Geometry check sheet. Reference: the model listing, model coordinates, mm. Face numbers are marked on the shaded views. A direction names the side the tool comes from. Give positions to 0.01 mm unless a question says otherwise; leave off trailing zeros. Write each loop counter-clockwise with the first axis right and the second up, starting at its lowest first coordinate (ties: lowest second). Pieces come first, ordered by that corner, then holes. Notation, with made-up numbers: M -6,28 L 24,28 A25 ccw 24,42 Z; hole C -9.5,85.25 d4. An arc over 180 degrees is marked long. Write each question's results on one line, items separated by ' | '.
```python
from build123d import *

# Parameters (mm, degrees)
SKETCH019_W             = 83
SKETCH019_H             = 28
SKETCH019_W_2           = 79
SKETCH019_H_2           = 24
REVOLUTION_ANGLE        = 35
SKETCH020_W             = 83
SKETCH020_H             = 28
SKETCH020_W_2           = 79
SKETCH020_H_2           = 24
PAD010_DEPTH            = 60
POCKET006_DEPTH         = 83.001
SKETCH022_W             = 83
SKETCH022_H             = 28
SKETCH022_W_2           = 79
SKETCH022_H_2           = 24
PAD011_DEPTH            = 15
BODY005_PLACEMENT_ANGLE = 180


with BuildPart() as part:
    # Sketch019 → Revolution (revolve)
    with BuildSketch(Plane(origin=(310, 156, 1), x_dir=(0, 1, 0), z_dir=(1, 0, 0))):
        with Locations((41.5, 14)):
            Rectangle(SKETCH019_W, SKETCH019_H)
        with Locations((41.5, 14)):
            Rectangle(SKETCH019_W_2, SKETCH019_H_2, mode=Mode.SUBTRACT)
    revolve(axis=Axis((310, 156, 1), (0, 1, 0)), revolution_arc=REVOLUTION_ANGLE)

    # Sketch020 (on Face9 of Revolution) → Pad010 (new body)
    with BuildSketch(Plane(origin=(207.543276, 0, -145.323366), x_dir=(0, 1, 0), z_dir=(0.819152, 0, -0.573576))):
        with Locations((197.5, 192.627847)):
            Rectangle(SKETCH020_W, SKETCH020_H)
        with Locations((197.5, 192.627847)):
            Rectangle(SKETCH020_W_2, SKETCH020_H_2, mode=Mode.SUBTRACT)
    extrude(amount=PAD010_DEPTH)

    # Sketch021 (on Face11 of Pad010) → Pocket006 (cut, through all)
    with BuildSketch(Plane(origin=(0, 156, 0), x_dir=(0, 0, -1), z_dir=(0, -1, 0))):
        Polygon((21.946458, 367.179193), (33.414586, 359.149123), (25.384516, 347.680994), align=None)
    extrude(amount=-POCKET006_DEPTH, mode=Mode.SUBTRACT)

    # Sketch022 (on Face4 of Pocket006) → Pad011 (join)
    with BuildSketch(Plane(origin=(310, 0, 0), x_dir=(0, 1, 0), z_dir=(-1, 0, 0))):
        with Locations((197.5, -15)):
            Rectangle(SKETCH022_W, SKETCH022_H)
        with Locations((197.5, -15)):
            Rectangle(SKETCH022_W_2, SKETCH022_H_2, mode=Mode.SUBTRACT)
    extrude(amount=PAD011_DEPTH)


with BuildPart() as part_1:
    # Body005 placement: moved
    add(part.part.moved(Location((0, 395, 30))).rotate(Axis((0, 395, 30), (1, 0, 0)), BODY005_PLACEMENT_ANGLE))


solid = part_1.part
```
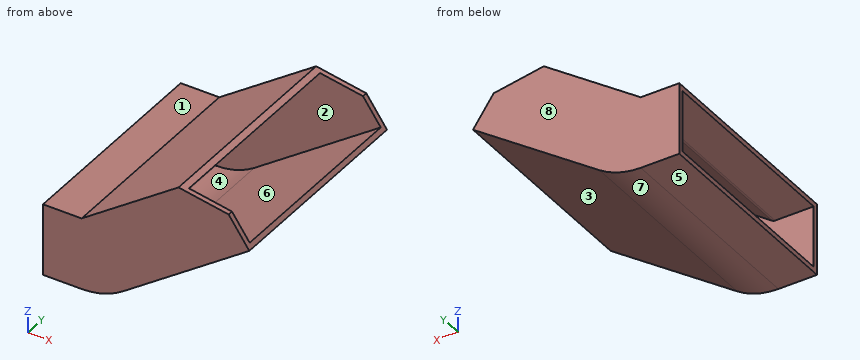
Q1. Section check C-C (z = 37.5). Enter the section's corners in (x, y).
Answer key:
outline: M 322.14,156 L 370.96,156 L 370.96,239 L 322.14,239 Z; hole M 325.63,158 L 367.47,158 L 367.47,237 L 325.63,237 Z
Q2. Access from +Z, -Z, +X, -X, +Y, -Y to the whole of each face (thin tool, end or side, straight path). Record for the marked faces 1, 2, 3, 4 and 5.
Answer key:
face 1: +Z, -X, +Y, -Y | face 2: none | face 3: -Z, +X, +Y, -Y | face 4: -X | face 5: -Z, +X, -X, +Y, -Y
Q3. Section check D-D (x = 368.5). Enter the section's corners in (y, z).
Answer key:
outline: M 156,35.78 L 239,35.78 L 239,50.06 L 237,50.06 L 237,38.22 L 158,38.22 L 158,50.06 L 156,50.06 Z
Q4. Release check for a two-part mould opening along X. For the marked faces 6, 7 and 8 record: released by +X, released by -X, zero draft, split by the parting line, or undercut.
Answer key:
face 6: undercut | face 7: released by +X | face 8: zero draft
Q5. Section check A-A (y = 191). Enter the section's corners in (x, z).
Answer key:
outline: M 295,1 L 310,1 A28 ccw 326.06,6.06 L 375.21,40.48 L 374.06,42.12 L 324.91,7.7 A26 cw 310,3 L 295,3 Z; M 295,27 L 310,27 A2 ccw 311.15,27.36 L 350.47,54.89 L 347.68,55.38 L 310,29 L 295,29 Z
Q6. Section check B-B (x = 315). Enter the section's corners in (y, z), then the cut area to 3 significant figures.
Answer key:
outline: M 156,1.45 L 239,1.45 L 239,32.5 L 156,32.5 Z; hole M 158,3.49 L 237,3.49 L 237,30.06 L 158,30.06 Z | area: 478 mm2
Q7. Depth check by flat-ended pin: P1, Ø6, axis at x = 331, y = 181.5, coming from the -Z side; P2, Ø10, axis at y = 167, z = 29.5, coming from the +X side; P3, Ø12, axis at y = 218.5, z = 15, coming from the +X side. Enter the tip coordinate at first touch or a pass-through.
Answer key:
P1: stops at z = 7.42 | P2: stops at x = 366.67 | P3: stops at x = 347.39
Q8. Material ranges on probe 1 along Y at (x, z) = (360.5, 45); probe 2 along Z at (x, y) = (298, 210); probe 3 along Z at (x, y) = (317, 169), recorded low to high. Write a range as [from, to].
Answer key:
probe 1: y = [156, 158], [237, 239] | probe 2: z = [1, 3], [27, 29] | probe 3: z = [1.89, 3.96], [31.46, 33.9]
